CAD build for the part. Positions are in the model's coordinates, mm. Round coordinates to 2 decimals unless told otherwise and drop trailing zeros. Loops run counter-clockwise (first coordinate to the right, second up) from the corner with the lowest first, then second, coordinate; pieces in that order, holes last. Notation, with made-up numbers: (89, -23) - (148, -23) arc R30 ccw to (148, 1) - close; hole circle Ø11 at (-16, 25). An arc over 180 degrees is marked (long way). Use one line per item in the form item = value.
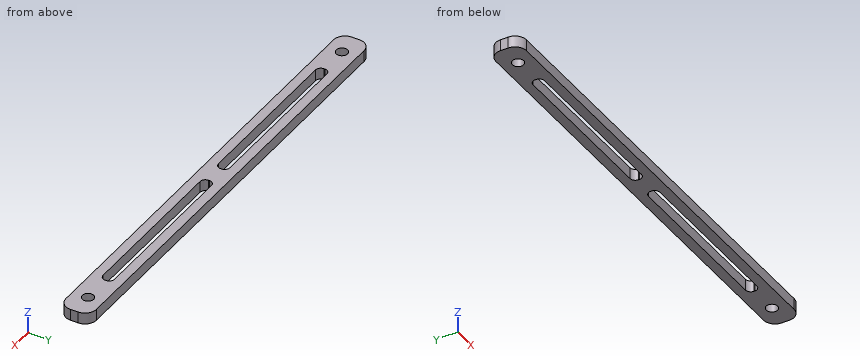
from build123d import *

# Parameters (mm, degrees)
SKETCH1_R           = 1.5
BOSS_EXTRUDE1_DEPTH = 3


with BuildPart() as part:
    # Sketch1 → Boss-Extrude1 (new body)
    with BuildSketch(Plane.XY):
        with BuildLine():
            Line((-58, 4), (58, 4))
            ThreePointArc((58, 4), (60.121320344, 3.121320344), (61, 1))
            Line((61, 1), (61, -1))
            ThreePointArc((61, -1), (60.121320344, -3.121320344), (58, -4))
            Line((58, -4), (-58, -4))
            ThreePointArc((-58, -4), (-60.121320344, -3.121320344), (-61, -1))
            Line((-61, -1), (-61, 1))
            ThreePointArc((-61, 1), (-60.121320344, 3.121320344), (-58, 4))
        make_face()
        with Locations((-55, 0)):
            Circle(SKETCH1_R, mode=Mode.SUBTRACT)
        with Locations((55, 0)):
            Circle(SKETCH1_R, mode=Mode.SUBTRACT)
        with BuildLine():
            Line((-46, 1.5), (-4, 1.5))
            ThreePointArc((-4, 1.5), (-3.010050506, 1.089949494), (-2.6, 0.1))
            Line((-2.6, 0.1), (-2.6, -0.1))
            ThreePointArc((-2.6, -0.1), (-3.010050506, -1.089949494), (-4, -1.5))
            Line((-4, -1.5), (-46, -1.5))
            ThreePointArc((-46, -1.5), (-46.989949494, -1.089949494), (-47.4, -0.1))
            Line((-47.4, -0.1), (-47.4, 0.1))
            ThreePointArc((-47.4, 0.1), (-46.989949494, 1.089949494), (-46, 1.5))
        make_face(mode=Mode.SUBTRACT)
        with BuildLine():
            Line((4, 1.494330249), (46, 1.494330249))
            ThreePointArc((46, 1.494330249), (46.989949494, 1.084279743), (47.4, 0.094330249))
            Line((47.4, 0.094330249), (47.4, -0.094330249))
            ThreePointArc((47.4, -0.094330249), (46.989949494, -1.084279743), (46, -1.494330249))
            Line((46, -1.494330249), (4, -1.494330249))
            ThreePointArc((4, -1.494330249), (3.010050506, -1.084279743), (2.6, -0.094330249))
            Line((2.6, -0.094330249), (2.6, 0.094330249))
            ThreePointArc((2.6, 0.094330249), (3.010050506, 1.084279743), (4, 1.494330249))
        make_face(mode=Mode.SUBTRACT)
    extrude(amount=BOSS_EXTRUDE1_DEPTH)


solid = part.part
1) Slice it at B-B (z = 0.65). Write the cut outline in (x, y).
Report:
outline = (-61, -1) arc R3 ccw to (-58, -4) - (58, -4) arc R3 ccw to (61, -1) - (61, 1) arc R3 ccw to (58, 4) - (-58, 4) arc R3 ccw to (-61, 1) - close; hole circle Ø3 at (-55, 0); hole (-47.4, -0.1) arc R1.4 ccw to (-46, -1.5) - (-4, -1.5) arc R1.4 ccw to (-2.6, -0.1) - (-2.6, 0.1) arc R1.4 ccw to (-4, 1.5) - (-46, 1.5) arc R1.4 ccw to (-47.4, 0.1) - close; hole (2.6, -0.09) arc R1.4 ccw to (4, -1.49) - (46, -1.49) arc R1.4 ccw to (47.4, -0.09) - (47.4, 0.09) arc R1.4 ccw to (46, 1.49) - (4, 1.49) arc R1.4 ccw to (2.6, 0.09) - close; hole circle Ø3 at (55, 0)
2) Slice it at A-A (x = 55). Write the cut outline in (y, z), plus the area to 3 significant figures.
Report:
outline = (-4, 0) - (-1.5, 0) - (-1.5, 3) - (-4, 3) - close; (1.5, 0) - (4, 0) - (4, 3) - (1.5, 3) - close
area = 15.0 mm^2
3) Slice it at C-C (x = 28). Write the cut outline in (y, z).
Report:
outline = (-4, 0) - (-1.49, 0) - (-1.49, 3) - (-4, 3) - close; (1.49, 0) - (4, 0) - (4, 3) - (1.49, 3) - close
4) Drill centre lines: probe 1 along X at (y, z) = (0.25, 1.15); probe 2 along Y at (x, z) = (-55, 0.9); probe 3 along X at (y, z) = (-2.5, 1.1). Where is each one in solid material? Low to high.
Report:
probe_1 = -61 to -56.48, -53.52 to -47.39, -2.61 to 2.61, 47.39 to 53.52, 56.48 to 61
probe_2 = -4 to -1.5, 1.5 to 4
probe_3 = -60.6 to 60.6
